Design review of the part built by this model. Coordinates are the model's own, in mm. A direction names the side the tool comes from. Round coordinates to 2 decimals unless told otherwise and drop trailing zeros. Order: outer loops, then holes, each group sorted by start corner. A loop starts at its lowest first (then second) coordinate and runs counter-clockwise, first axis right, second up. Notation, with made-up numbers: (34.25, 86.25) - (60.25, 86.25) arc R17 cw to (60.25, 114.25) - close; hole circle Ø2 at (1, -32.5). An arc over 180 degrees is marked (long way). Write item = value, one per line.
from build123d import *

# Parameters (mm, degrees)
ESQUISSE1_R        = 16.5
BOSS_EXTRU_1_DEPTH = 55
CHANFREIN1_SIZE    = 1


with BuildPart() as part:
    # Esquisse1 → Boss.-Extru.1 (new body)
    with BuildSketch(Plane(origin=(0, 0, 0), x_dir=(1, 0, 0), z_dir=(0, 1, 0))):
        with Locations(Location((0, 0, 0), (0, 0, 270))):  # turned: the seam where the file's is
            Circle(ESQUISSE1_R)
    extrude(amount=BOSS_EXTRU_1_DEPTH)

    # Esquisse5 → Révolution1 (revolve)
    with BuildSketch(Plane.XY, mode=Mode.PRIVATE) as r_volution1_sk:
        with BuildLine():
            Line((0, 55), (18.5, 55))
            ThreePointArc((18.5, 55), (16.5, 61), (18.5, 67))
            ThreePointArc((18.5, 67), (16.5, 73), (18.5, 79))
            ThreePointArc((18.5, 79), (16.5, 85), (18.5, 91))
            Line((18.5, 91), (18.5, 136))
            Line((18.5, 136), (0, 136))
            Line((0, 136), (0, 55))
        make_face()
    revolve(r_volution1_sk.sketch.rotate(Axis((0, 136, 0), (0, -1, 0)), 180), axis=Axis((0, 136, 0), (0, -1, 0)))  # turned: the seam where the file's is

    # Chanfrein1
    chanfrein1_edges = [part.edges().sort_by_distance(p)[0] for p in [
        (18.5, 136, 0),
    ]]
    chamfer(chanfrein1_edges, length=CHANFREIN1_SIZE)


solid = part.part
Item 1: Take a section at C-C, the plane y = 63. State the section outline as (x, z) points.
Data:
outline = circle Ø33.4 at (0, 0)
Item 2: Take a section at A-A, the plane x = 0. State the section outline as (y, z) points, and give its area (3 significant figures).
Data:
outline = (0, -16.5) - (55, -16.5) - (55, -18.5) arc R10 cw to (67, -18.5) arc R10 cw to (79, -18.5) arc R10 cw to (91, -18.5) - (135, -18.5) - (136, -17.5) - (136, 17.5) - (135, 18.5) - (91, 18.5) arc R10 cw to (79, 18.5) arc R10 cw to (67, 18.5) arc R10 cw to (55, 18.5) - (55, 16.5) - (0, 16.5) - close
area = 4,710 mm2
Item 3: For line 1 along X through (y, z) = (43, 0.5); line 2 along Z through (x, y) = (6, 108.5), list the stretches that pass through material, from the lowest coordinate up. Write a range as [from, to].
Data:
line_1 = [-16.49, 16.49]
line_2 = [-17.5, 17.5]
Item 4: For faces 1 (the face through (-16.108, 27.115, -3.577)), 2 (the face through (0, 0, 0)), list the 3-axis set-ups (+Z, -Z, +X, -X, +Y, -Y) from which the entire face can be reached by the end or side of a thin tool; tool diameter is ignored.
Data:
face_1 = -Y
face_2 = +Z, -Z, +X, -X, -Y
Item 5: Take a section at B-B, the plane y = 29.5. State the section outline as (x, z) points, and give its area (3 significant figures).
Data:
outline = circle Ø33 at (0, 0)
area = 855 mm2
Item 6: Insertion check: P1, Ø3, axis at y = 79.5, z = 4, coming from the +X side; P2, Ø1.5, axis at x = -6, z = -12, coming from the -Y side; P3, Ø5, axis at x = 11, y = 15, coming from the -Z side; P4, Ø4, axis at x = 1, y = 119.5, coming from the +Z side. Each pin has a flat end and moves straight along its axis. Give the tip position at first contact, or say it passes through.
Data:
P1 = 18.32
P2 = 0
P3 = -14.14
P4 = 18.5
